Input: part model. Units: mm. Frame: model coordinates. Face numbers are marked on the shaded views. A direction names the side the tool comes from. Round coordinates to 2 decimals unless told otherwise and drop trailing zeros. Loops run counter-clockwise (first coordinate to the right, second up) from the corner with the lowest first, then second, coordinate; pieces in that order, holes last. Notation, with made-up numbers: (-22.5, 49) - (1.5, 49) arc R26 ccw to (1.5, 65) - close; hole circle Ø7 at (2.25, 14.25). An arc over 180 degrees is marked (long way). One line per question, with ' | ' between items. Start each with the question number.
Item 1: Draft query along X for the marked faces 1, 2 and 3. Return one class per face: pulls with the +X half, pulls with the -X half, needs draft (parallel to the pull), parting line crosses it, or undercut.
Item 2: First-contact query: pin 1 (1.8 mm diameter, centred on x = -15.56, y = -15.56, fed in from -Z); pin 2 (1.5 mm diameter, centred on y = 22.5, z = 3, fed in from -X); pin 3 (3 mm diameter, centred on x = -15.5, z = 3, fed in from +Y); pin 4 (2 mm diameter, centred on x = 9.5, z = 2.5, fed in from -Y). Flat tips, straight axial feed; report the tip coordinate or a pass-through.
Item 3: Section C-C, the plane z = 3.65. Return loops of the section in (x, y), plus the area to 3 significant figures.
Item 4: Section A-A, the plane x = 0. Return loops of the section in (y, z).
Item 5: Set-up query: the marked faces 4 and 5. Return all of +Z, -Z, +X, -X, +Y, -Y with unobstructed straight access to the full face (end or side cutting, diameter ignored); none if empty.
Item 6: Material intervals for line 1 along Y through (x, z) = (15, 3.15); line 2 along X through (y, z) = (-14.5, 1.55); line 3 along X through (y, z) = (-8.5, 4.45), sorted ascending.
Item 7: Section B-B, the plane y = 11. Return loops of the section in (x, z), plus the area to 3 significant figures.
Item 8: Section D-D, the plane x = -26. Return loops of the section in (y, z).
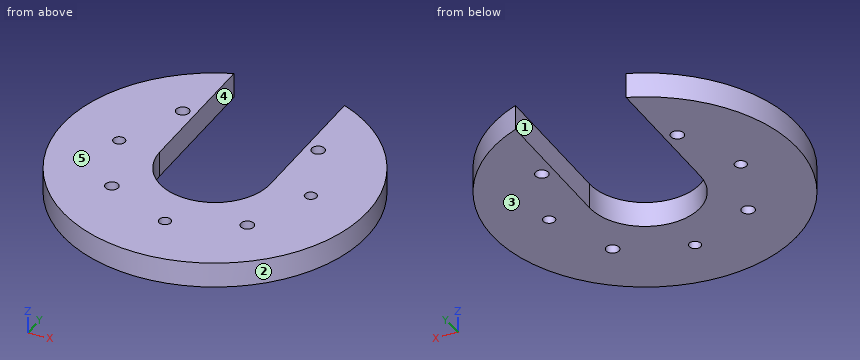
```python
from build123d import *

# Parameters (mm, degrees)
SKETCH1_R           = 1.35
BOSS_EXTRUDE1_DEPTH = 5.842
SKETCH2_R           = 1.5
CUT_EXTRUDE1_DEPTH  = 50.860559066


with BuildPart() as part:
    # Sketch1 → Boss-Extrude1 (new body)
    with BuildSketch(Plane.XY):
        with BuildLine():
            Line((-12.7, 0), (-12.7, 32.629483496))
            ThreePointArc((-12.7, 32.629483496), (0, -35.0139), (12.7, 32.629483496))
            Line((12.7, 32.629483496), (12.7, 0))
            ThreePointArc((12.7, 0), (0, -12.7), (-12.7, 0))
        make_face()
        with Locations((22, 0)):
            Circle(SKETCH1_R, mode=Mode.SUBTRACT)
        with Locations((0, -22)):
            Circle(SKETCH1_R, mode=Mode.SUBTRACT)
        with Locations((-22, 0)):
            Circle(SKETCH1_R, mode=Mode.SUBTRACT)
    extrude(amount=BOSS_EXTRUDE1_DEPTH)

    # Sketch2 → Cut-Extrude1 (cut, through all)
    with BuildSketch(Plane.XY.offset(5.842)):
        with Locations((-15.556349186, -15.556349186)):
            Circle(SKETCH2_R)
        with Locations((-15.556349186, 15.556349186)):
            Circle(SKETCH2_R)
        with Locations((15.556349186, 15.556349186)):
            Circle(SKETCH2_R)
        with Locations((15.556349186, -15.556349186)):
            Circle(SKETCH2_R)
    extrude(amount=-CUT_EXTRUDE1_DEPTH, mode=Mode.SUBTRACT)


solid = part.part
```
Return value:
1) face 1: undercut | face 2: parting line crosses it | face 3: needs draft
2) pin 1: through | pin 2: x = -27.44 | pin 3: y = 32.09 | pin 4: y = -33.97
3) outline: (-12.7, 0) - (-12.7, 32.63) arc R35.01 ccw (long way) to (12.7, 32.63) - (12.7, 0) arc R12.7 cw to start; hole circle Ø2.7 at (-22, 0); hole circle Ø3 at (-15.56, -15.56); hole circle Ø3 at (-15.56, 15.56); hole circle Ø2.7 at (0, -22); hole circle Ø3 at (15.56, -15.56); hole circle Ø3 at (15.56, 15.56); hole circle Ø2.7 at (22, 0) | area: 2,680 mm2
4) outline: (-35.01, 0) - (-23.35, 0) - (-23.35, 5.84) - (-35.01, 5.84) - close; (-20.65, 0) - (-12.7, 0) - (-12.7, 5.84) - (-20.65, 5.84) - close
5) face 4: +Z, -Z, +Y | face 5: +Z, +X, -X, +Y, -Y
6) line 1: -31.64 to -16.95, -14.16 to 14.16, 16.95 to 31.64 | line 2: -31.87 to -16.62, -14.49 to 14.49, 16.62 to 31.87 | line 3: -33.97 to -9.44, 9.44 to 33.97
7) outline: (-33.24, 0) - (-12.7, 0) - (-12.7, 5.84) - (-33.24, 5.84) - close; (12.7, 0) - (33.24, 0) - (33.24, 5.84) - (12.7, 5.84) - close | area: 240 mm2
8) outline: (-23.45, 0) - (23.45, 0) - (23.45, 5.84) - (-23.45, 5.84) - close
